Part model, mm, in its own coordinate system. A direction names the side the tool comes from. Round coordinates to 2 decimals unless told otherwise and drop trailing zeros. Loops run counter-clockwise (first coordinate to the right, second up) from the corner with the lowest first, then second, coordinate; pieces in that order, holes last. Notation, with made-up numbers: M 24.5,-39.75 L 39.5,-39.75 A33 cw 39.5,-5.75 Z; hole C 32.5,67.25 d7. An arc over 180 degrees is marked long. Put each result on its own line as item: value. Start each with the question number.
1) Slice it at A-A on x = 13. Give the cut face in (y, z).
2) Slice it at D-D on x = 58.5. Give the cut face in (y, z).
3) Slice it at C-C on z = 8.25. Give the cut face in (x, y), then the cut area to 3 significant figures.
4) Probe line 1 along Y through (x, z) = (39.5, 2.9); line 2 along Y through (x, z) = (125, 1.6); line 3 along X through (y, z) = (31.5, 4.5). List the from-to ranges inside material, lowest first.
5) Pull direction Y, two halves, no side cores. Call faces 5 (the flat face through (113, 42.5, 3)), 6 (the flat face through (66, 22, 5)), 7 (the cylindrical face through (93.408, 36.756, 2.465)): +Y half, -Y half, draft (parallel to the pull), parting line (faces both ways), or undercut.
6) Drop flat-ended pins along their axis: pin 1 Ø2.5 at (x, y) = (100, 39) entering from +Z; pin 2 Ø3 at (y, z) = (54, 6.5) entering from -X; pin 3 Ø1.5 at (x, y) = (116.5, 26.5) entering from +Z; pin 4 Ø2 at (x, y) = (9, 59.5) entering from +Z. Give the stop position or say it passes through.
7) Which spindle directions (+Z, -Z, +X, -X, +Y, -Y) get a long thin tool onto all of the face, cutting with end or side? Do faces 1 (the flat face through (77, 41, 0)), 2 (the flat face through (113, 24.5, 3)), 3 (the flat face through (24, 58, 2)), 4 (the cylindrical face through (115, 7, 8)). Say none if no direction does.
8) Slice it at B-B on y = 18. State how many separate pieces and enclosed holes the cut face has, then the cut area to 3 significant figures.
```python
from build123d import *

# Parameters (mm, degrees)
BOX_W             = 128
BOX_H             = 67
BOX_DEPTH         = 2
BOX001_W          = 37
BOX001_H          = 60
BOX001_DEPTH      = 2
BOX002_W          = 35
BOX002_H          = 49
BOX002_DEPTH      = 4
BOX003_W          = 78
BOX003_H          = 23
BOX003_DEPTH      = 1
BOX004_W          = 40
BOX004_H          = 40
BOX004_DEPTH      = 3
CYLINDER_R        = 17.5
CYLINDER_DEPTH    = 5
CYLINDER001_R     = 1.5
CYLINDER001_DEPTH = 3
CYLINDER002_R     = 1.5
CYLINDER002_DEPTH = 3
CYLINDER003_R     = 1.5
CYLINDER003_DEPTH = 3
CYLINDER004_R     = 1.5
CYLINDER004_DEPTH = 3
BOX005_W          = 18
BOX005_H          = 18
BOX005_DEPTH      = 3
CYLINDER005_R     = 1.5
CYLINDER005_DEPTH = 3
CYLINDER006_R     = 1.5
CYLINDER006_DEPTH = 3
CYLINDER007_R     = 3
CYLINDER007_DEPTH = 9
CYLINDER008_R     = 1.5
CYLINDER008_DEPTH = 5
CYLINDER009_R     = 3
CYLINDER009_DEPTH = 9
CYLINDER010_R     = 1.5
CYLINDER010_DEPTH = 5
BOX006_W          = 10
BOX006_H          = 25
BOX006_DEPTH      = 1.5
BOX007_W          = 4
BOX007_H          = 7
BOX007_DEPTH      = 6
CYLINDER011_R     = 1.5
CYLINDER011_DEPTH = 2.5
CYLINDER012_R     = 1.5
CYLINDER012_DEPTH = 2.5
CYLINDER013_R     = 1
CYLINDER013_DEPTH = 2
CYLINDER014_R     = 1
CYLINDER014_DEPTH = 2
CYLINDER015_R     = 1
CYLINDER015_DEPTH = 2
CYLINDER016_R     = 1
CYLINDER016_DEPTH = 2
CYLINDER017_R     = 1.25
CYLINDER017_DEPTH = 2
CYLINDER018_R     = 1.25
CYLINDER018_DEPTH = 2
CYLINDER019_R     = 1.25
CYLINDER019_DEPTH = 2
CYLINDER020_R     = 1.25
CYLINDER020_DEPTH = 2
FILLET_R          = 1.5


with BuildPart() as part:
    # Box → Box (join)
    with BuildSketch(Plane.XY):
        with Locations((64, 33.5)):
            Rectangle(BOX_W, BOX_H)
    extrude(amount=BOX_DEPTH)

    # Box001 → Box001 (join)
    with BuildSketch(Plane(origin=(6, 3.5, 2), x_dir=(1, 0, 0), z_dir=(0, 0, 1))):
        with Locations((18.5, 30)):
            Rectangle(BOX001_W, BOX001_H)
    extrude(amount=BOX001_DEPTH)

    # Box002 → Box002 (cut)
    with BuildSketch(Plane(origin=(7, 9, 0), x_dir=(1, 0, 0), z_dir=(0, 0, 1))):
        with Locations((17.5, 24.5)):
            Rectangle(BOX002_W, BOX002_H)
    extrude(amount=BOX002_DEPTH, mode=Mode.SUBTRACT)

    # Box003 → Box003 (cut)
    with BuildSketch(Plane(origin=(44, 42, 1), x_dir=(1, 0, 0), z_dir=(0, 0, 1))):
        with Locations((39, 11.5)):
            Rectangle(BOX003_W, BOX003_H)
    extrude(amount=BOX003_DEPTH, mode=Mode.SUBTRACT)

    # Box004 → Box004 (join)
    with BuildSketch(Plane(origin=(64, 2, 2), x_dir=(1, 0, 0), z_dir=(0, 0, 1))):
        with Locations((20, 20)):
            Rectangle(BOX004_W, BOX004_H)
    extrude(amount=BOX004_DEPTH)

    # Cylinder → Cylinder (cut)
    with BuildSketch(Plane(origin=(84, 22, 0), x_dir=(1, 0, 0), z_dir=(0, 0, 1))):
        Circle(CYLINDER_R)
    extrude(amount=CYLINDER_DEPTH, mode=Mode.SUBTRACT)

    # Cylinder001 → Cylinder001 (cut)
    with BuildSketch(Plane(origin=(67.5, 5.5, 2), x_dir=(1, 0, 0), z_dir=(0, 0, 1))):
        Circle(CYLINDER001_R)
    extrude(amount=CYLINDER001_DEPTH, mode=Mode.SUBTRACT)

    # Cylinder002 → Cylinder002 (cut)
    with BuildSketch(Plane(origin=(67.5, 38.5, 2), x_dir=(1, 0, 0), z_dir=(0, 0, 1))):
        Circle(CYLINDER002_R)
    extrude(amount=CYLINDER002_DEPTH, mode=Mode.SUBTRACT)

    # Cylinder003 → Cylinder003 (cut)
    with BuildSketch(Plane(origin=(100.5, 38.5, 2), x_dir=(1, 0, 0), z_dir=(0, 0, 1))):
        Circle(CYLINDER003_R)
    extrude(amount=CYLINDER003_DEPTH, mode=Mode.SUBTRACT)

    # Cylinder004 → Cylinder004 (cut)
    with BuildSketch(Plane(origin=(100.5, 5.5, 2), x_dir=(1, 0, 0), z_dir=(0, 0, 1))):
        Circle(CYLINDER004_R)
    extrude(amount=CYLINDER004_DEPTH, mode=Mode.SUBTRACT)

    # Box005 → Box005 (join)
    with BuildSketch(Plane(origin=(110, 24.5, 2), x_dir=(1, 0, 0), z_dir=(0, 0, 1))):
        with Locations((9, 9)):
            Rectangle(BOX005_W, BOX005_H)
    extrude(amount=BOX005_DEPTH)

    # Cylinder005 → Cylinder005 (cut)
    with BuildSketch(Plane(origin=(116.5, 26, 2), x_dir=(1, 0, 0), z_dir=(0, 0, 1))):
        Circle(CYLINDER005_R)
    extrude(amount=CYLINDER005_DEPTH, mode=Mode.SUBTRACT)

    # Cylinder006 → Cylinder006 (cut)
    with BuildSketch(Plane(origin=(116.5, 41, 2), x_dir=(1, 0, 0), z_dir=(0, 0, 1))):
        Circle(CYLINDER006_R)
    extrude(amount=CYLINDER006_DEPTH, mode=Mode.SUBTRACT)

    # Cylinder007 → Cylinder007 (join)
    with BuildSketch(Plane(origin=(116.5, 7, 2), x_dir=(1, 0, 0), z_dir=(0, 0, 1))):
        Circle(CYLINDER007_R)
    extrude(amount=CYLINDER007_DEPTH)

    # Cylinder008 → Cylinder008 (cut)
    with BuildSketch(Plane(origin=(116.5, 7, 6), x_dir=(1, 0, 0), z_dir=(0, 0, 1))):
        Circle(CYLINDER008_R)
    extrude(amount=CYLINDER008_DEPTH, mode=Mode.SUBTRACT)

    # Cylinder009 → Cylinder009 (join)
    with BuildSketch(Plane(origin=(58.5, 7, 2), x_dir=(1, 0, 0), z_dir=(0, 0, 1))):
        Circle(CYLINDER009_R)
    extrude(amount=CYLINDER009_DEPTH)

    # Cylinder010 → Cylinder010 (cut)
    with BuildSketch(Plane(origin=(58.5, 7, 6), x_dir=(1, 0, 0), z_dir=(0, 0, 1))):
        Circle(CYLINDER010_R)
    extrude(amount=CYLINDER010_DEPTH, mode=Mode.SUBTRACT)

    # Box006 → Box006 (join)
    with BuildSketch(Plane(origin=(46.5, 12, 2), x_dir=(1, 0, 0), z_dir=(0, 0, 1))):
        with Locations((5, 12.5)):
            Rectangle(BOX006_W, BOX006_H)
    extrude(amount=BOX006_DEPTH)

    # Box007 → Box007 (cut)
    with BuildSketch(Plane(origin=(49.5, 21, -1.5), x_dir=(1, 0, 0), z_dir=(0, 0, 1))):
        with Locations((2, 3.5)):
            Rectangle(BOX007_W, BOX007_H)
    extrude(amount=BOX007_DEPTH, mode=Mode.SUBTRACT)

    # Cylinder011 → Cylinder011 (cut)
    with BuildSketch(Plane(origin=(51.5, 18, 1), x_dir=(1, 0, 0), z_dir=(0, 0, 1))):
        Circle(CYLINDER011_R)
    extrude(amount=CYLINDER011_DEPTH, mode=Mode.SUBTRACT)

    # Cylinder012 → Cylinder012 (cut)
    with BuildSketch(Plane(origin=(51.5, 32, 1), x_dir=(1, 0, 0), z_dir=(0, 0, 1))):
        Circle(CYLINDER012_R)
    extrude(amount=CYLINDER012_DEPTH, mode=Mode.SUBTRACT)

    # Cylinder013 → Cylinder013 (cut)
    with BuildSketch(Plane(origin=(9.5, 7, 2), x_dir=(1, 0, 0), z_dir=(0, 0, 1))):
        Circle(CYLINDER013_R)
    extrude(amount=CYLINDER013_DEPTH, mode=Mode.SUBTRACT)

    # Cylinder014 → Cylinder014 (cut)
    with BuildSketch(Plane(origin=(9.5, 60, 2), x_dir=(1, 0, 0), z_dir=(0, 0, 1))):
        Circle(CYLINDER014_R)
    extrude(amount=CYLINDER014_DEPTH, mode=Mode.SUBTRACT)

    # Cylinder015 → Cylinder015 (cut)
    with BuildSketch(Plane(origin=(39.5, 60, 2), x_dir=(1, 0, 0), z_dir=(0, 0, 1))):
        Circle(CYLINDER015_R)
    extrude(amount=CYLINDER015_DEPTH, mode=Mode.SUBTRACT)

    # Cylinder016 → Cylinder016 (cut)
    with BuildSketch(Plane(origin=(39.5, 7, 2), x_dir=(1, 0, 0), z_dir=(0, 0, 1))):
        Circle(CYLINDER016_R)
    extrude(amount=CYLINDER016_DEPTH, mode=Mode.SUBTRACT)

    # Cylinder017 → Cylinder017 (cut)
    with BuildSketch(Plane(origin=(3, 3, 0), x_dir=(1, 0, 0), z_dir=(0, 0, 1))):
        Circle(CYLINDER017_R)
    extrude(amount=CYLINDER017_DEPTH, mode=Mode.SUBTRACT)

    # Cylinder018 → Cylinder018 (cut)
    with BuildSketch(Plane(origin=(3, 64, 0), x_dir=(1, 0, 0), z_dir=(0, 0, 1))):
        Circle(CYLINDER018_R)
    extrude(amount=CYLINDER018_DEPTH, mode=Mode.SUBTRACT)

    # Cylinder019 → Cylinder019 (cut)
    with BuildSketch(Plane(origin=(125, 64, 0), x_dir=(1, 0, 0), z_dir=(0, 0, 1))):
        Circle(CYLINDER019_R)
    extrude(amount=CYLINDER019_DEPTH, mode=Mode.SUBTRACT)

    # Cylinder020 → Cylinder020 (cut)
    with BuildSketch(Plane(origin=(125, 3, 0), x_dir=(1, 0, 0), z_dir=(0, 0, 1))):
        Circle(CYLINDER020_R)
    extrude(amount=CYLINDER020_DEPTH, mode=Mode.SUBTRACT)

    # Fillet
    fillet_edges = [part.edges().sort_by_distance(p)[0] for p in [
        (64, 0, 0),
        (0, 33.5, 0),
        (64, 67, 0),
        (128, 33.5, 0),
    ]]
    fillet(fillet_edges, radius=FILLET_R)


solid = part.part
```
Recorded:
1. outline: M 0,1.5 A1.5 ccw 1.5,0 L 9,0 L 9,4 L 3.5,4 L 3.5,2 L 0,2 Z; M 58,0 L 65.5,0 A1.5 ccw 67,1.5 L 67,2 L 63.5,2 L 63.5,4 L 58,4 Z
2. outline: M 0,1.5 A1.5 ccw 1.5,0 L 65.5,0 A1.5 ccw 67,1.5 L 67,2 L 65,2 L 65,1 L 42,1 L 42,2 L 10,2 L 10,11 L 8.5,11 L 8.5,6 L 5.5,6 L 5.5,11 L 4,11 L 4,2 L 0,2 Z
3. outline: C 58.5,7 d6; C 116.5,7 d6; hole C 58.5,7 d3; hole C 116.5,7 d3
3. area: 42.4 mm2
4. line 1: y = 3.5 to 6, 8 to 9, 58 to 59, 61 to 63.5
4. line 2: y = 0 to 1.75, 4.25 to 62.75, 65.25 to 67
4. line 3: x = 64 to 69.3, 98.7 to 104, 110 to 128
5. face 5: +Y half
5. face 6: draft
5. face 7: undercut
6. pin 1: stops at z = 5
6. pin 2: passes through
6. pin 3: stops at z = 2
6. pin 4: stops at z = 4
7. face 1: -Z, +X, -X, +Y, -Y
7. face 2: +Z, +X
7. face 3: +Z, -Z
7. face 4: +Z
8. separate pieces: 3
8. enclosed holes: 0
8. area: 146 mm2
